```python
from build123d import *

# Parameters (mm, degrees)
F0_R     = 11.1125
F0_R_2   = 3.175
F1_DEPTH = 15.875
F2_R     = 4.7625
F2_R_2   = 3.175
F3_DEPTH = 2.54
F4_R     = 1.27
F5_DEPTH = 11.1135


with BuildPart() as f1:
    # F0 (on Front) → F1 (new body)
    with BuildSketch(Plane.XZ):
        Circle(F0_R)
        Circle(F0_R_2, mode=Mode.SUBTRACT)
    extrude(amount=F1_DEPTH)

    # F2 (on face) → F3 (cut)
    with BuildSketch(Plane.XZ.offset(15.875)):
        Circle(F2_R)
        Circle(F2_R_2, mode=Mode.SUBTRACT)
    extrude(amount=-F3_DEPTH, mode=Mode.SUBTRACT)

    # F4 (on Right) → F5 (cut, through all)
    with BuildSketch(Plane.YZ):
        with Locations((-6.985, 0)):
            Circle(F4_R)
    extrude(amount=F5_DEPTH, mode=Mode.SUBTRACT)


solid = f1.part
```
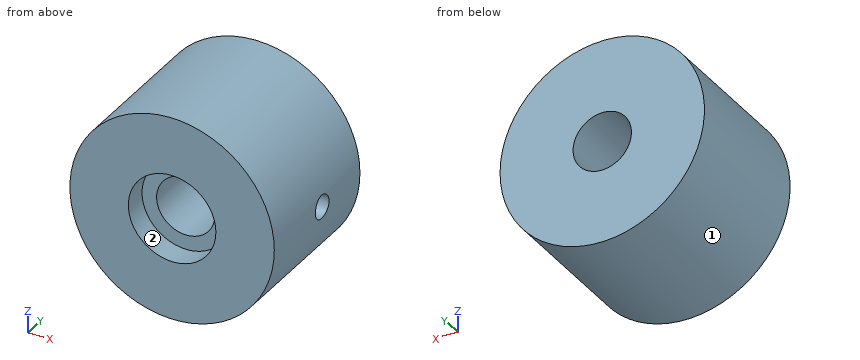
Geometry: final body of the model. Coordinates: model frame, mm. Face numbers are marked on the shaded views. A direction names the side the tool comes from. Round coordinates to 2 decimals unless told otherwise and drop trailing zeros. Write each loop counter-clockwise with the first axis right and the second up, starting at its lowest first coordinate (ties: lowest second). Pieces come first, ordered by that corner, then holes.
Item 1: Pin query (flat end, axial travel): P1, Ø1, axis at y = -6.5, z = -6, coming from the -X side; P2, Ø4, axis at x = -8.5, y = -4.5, coming from the +Z side; P3, Ø1.5, axis at y = -13.5, z = -2.5, coming from the -X side; P4, Ø11, axis at x = 0, z = 0, coming from the -Y side (3 decimals). Return the tip coordinate at first contact, or that it passes through.
Item 2: Section query C-C (x = 9). Return loops of the section in (y, z) (3 decimals), plus the area to 3 significant figures.
Item 3: Section query B-B (x = 0). Return loops of the section in (y, z) (1 decimal).
Item 4: Section query A-A (z = 0). Return loops of the section in (x, y) (1 decimal), plus the area to 3 significant figures.
Item 5: Material intervals for L1, parallel to Y at x = 7, z = 0 (3 decimals); L2, parallel to Z at x = 0, y = -13.9; L3, parallel to Y at x = 2, z = 3.5 (3 decimals), sorted ascending.
Item 6: Set-up query: the marked faces 1 and 2. Return all of +Z, -Z, +X, -X, +Y, -Y with unobstructed straight access to the full face (end or side cutting, diameter ignored); none if empty.
Completed:
1. P1: stops at x = -9.66
1. P2: stops at z = 9.01
1. P3: stops at x = -10.97
1. P4: stops at y = -15.875
2. outline: (-15.875, -6.518) - (0, -6.518) - (0, 6.518) - (-15.875, 6.518) - close; hole circle Ø2.54 at (-6.985, 0)
2. area: 202 mm2
3. outline: (-15.9, -11.1) - (0, -11.1) - (0, -3.2) - (-13.3, -3.2) - (-13.3, -4.8) - (-15.9, -4.8) - close; (-15.9, 4.8) - (-13.3, 4.8) - (-13.3, 3.2) - (0, 3.2) - (0, 11.1) - (-15.9, 11.1) - close
4. outline: (-11.1, -15.9) - (-4.8, -15.9) - (-4.8, -13.3) - (-3.2, -13.3) - (-3.2, 0) - (-11.1, 0) - close; (3.2, -13.3) - (4.8, -13.3) - (4.8, -15.9) - (11.1, -15.9) - (11.1, -8.3) - (3.2, -8.3) - close; (3.2, -5.7) - (11.1, -5.7) - (11.1, 0) - (3.2, 0) - close
4. area: 224 mm2
5. L1: y = -15.875 to -8.255, -5.715 to 0
5. L2: z = -11.11 to -4.76, 4.76 to 11.11
5. L3: y = -13.335 to 0
6. face 1: +Y, -Y
6. face 2: -Y
